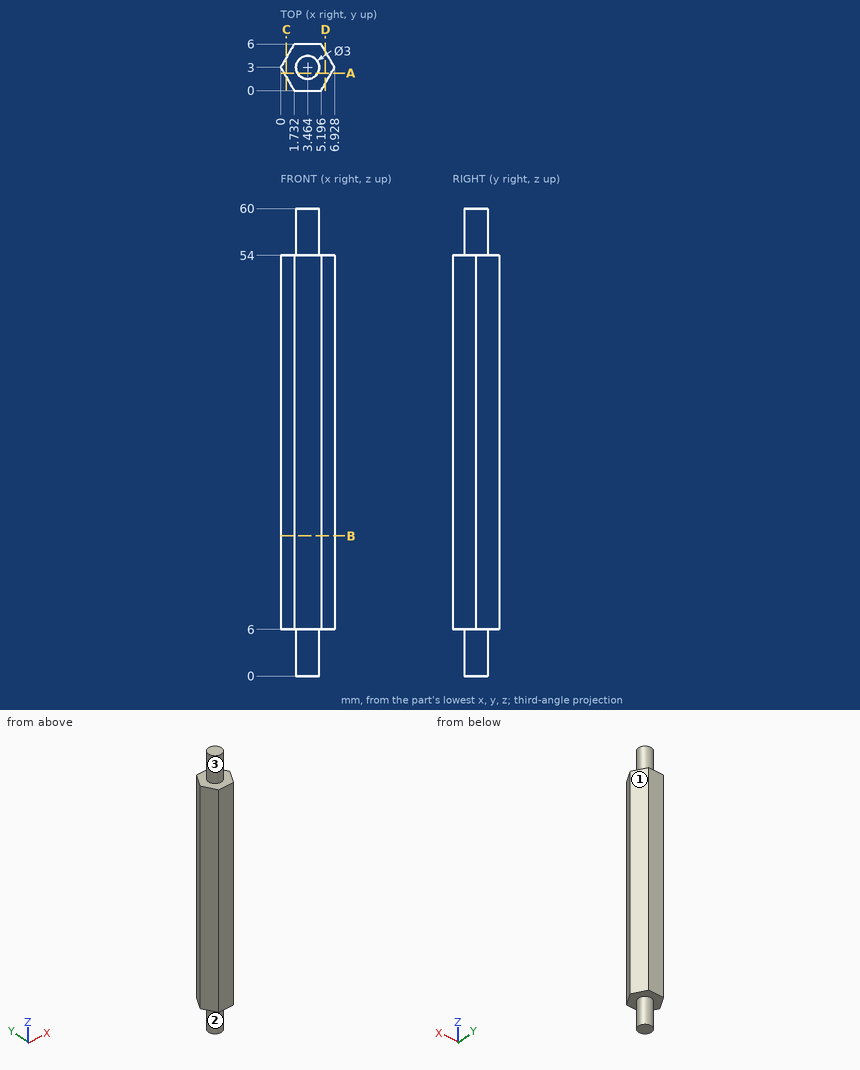
Could you check a few things on this drawing? It's one solid part, dimensions in mm from its lowest x, y, z. A direction names the side the tool comes from. Give positions to 0.01 mm unless a question says otherwise; leave off trailing zeros. Write each loop counter-clockwise with the first axis right and the second up, starting at its lowest first coordinate (ties: lowest second). Pieces come first, ordered by that corner, then holes. Notation, with made-up numbers: (33, 7.5) - (49, 7.5) arc R27 cw to (49, 38.5) - close; hole circle Ø4 at (84, -20). An arc over 180 degrees is marked (long way). Use CSV: the item, a comma, the result in double quotes. Start each with the question number.
Item 1: I want a section at C-C, the plane x = 0.75. Please give me the cut outline in (y, z).
Item 2: I want a section at B-B, the plane z = 18. Please give me the cut outline in (x, y), then the cut area to 3 significant figures.
Item 3: For the marked faces 1, 2 and 3, which set-ups out of +Z, -Z, +X, -X, +Y, -Y let a thin tool reach every point of the face, with its end or its side?
Item 4: I'm going to push a flat-ended pin straight in: pin 1 (3 mm diameter, centred on x = 4, y = 2.5, fed in from -Z). Where does the tip first touch, or does it pass through?
Item 5: I want a section at D-D, the plane x = 5.75. Please give me the cut outline in (y, z), then the cut area to 3 significant figures.
Item 6: If I drill on line 1 along Z through (x, y) = (5.5, 4); line 2 along Y through (x, z) = (6.75, 25); line 3 along Y through (x, z) = (5.75, 23), over which ranges is the centre line in solid material (lowest first)?
Item 7: I want a section at A-A, the plane y = 2.25. Please give me the cut outline in (x, z) (1 decimal), then the cut area to 3 significant figures.
Findings:
1,outline,"(1.7, 6) - (4.3, 6) - (4.3, 54) - (1.7, 54) - close"
2,outline,"(0, 3) - (1.73, 0) - (5.2, 0) - (6.93, 3) - (5.2, 6) - (1.73, 6) - close"
2,area,"31.2 mm2"
3,face 1,"+Z, -Z, +X, +Y"
3,face 2,"-Z"
3,face 3,"+Z"
4,pin 1,"stops at z = 0"
5,outline,"(0.96, 6) - (5.04, 6) - (5.04, 54) - (0.96, 54) - close"
5,area,"196 mm2"
6,line 1,"z = 6 to 54"
6,line 2,"y = 2.69 to 3.31"
6,line 3,"y = 0.96 to 5.04"
7,outline,"(0.4, 6) - (2.2, 6) - (2.2, 0) - (4.8, 0) - (4.8, 6) - (6.5, 6) - (6.5, 54) - (4.8, 54) - (4.8, 60) - (2.2, 60) - (2.2, 54) - (0.4, 54) - close"
7,area,"322 mm2"
